Geometry: final body of the model. Coordinates: model frame, mm. Face numbers are marked on the shaded views. A direction names the side the tool comes from. Round coordinates to 2 decimals unless told otherwise and drop trailing zeros. Loops run counter-clockwise (first coordinate to the right, second up) from the corner with the lowest first, then second, coordinate; pieces in that order, holes last. Notation, with made-up numbers: (13, -20) - (62, -20) arc R20 cw to (62, 4) - close; hole circle Ø11 at (68.25, 36.5). An arc over 180 degrees is marked (long way). Answer as CSV lines item,"result".
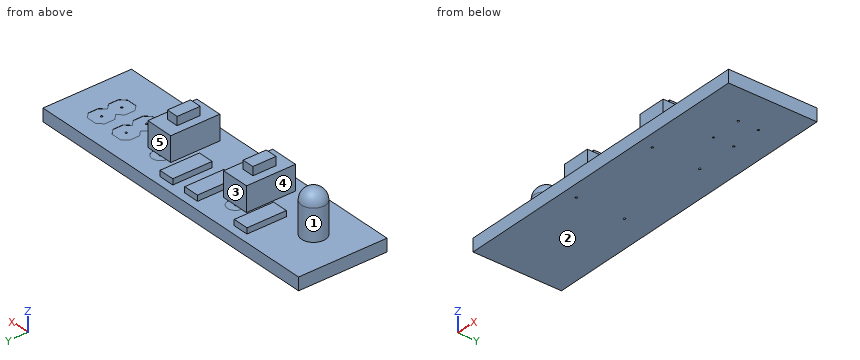
from build123d import *

# Parameters (mm, degrees)
SKETCH2_W           = 39.35
SKETCH2_H           = 11.1
BOSS_EXTRUDE1_DEPTH = 1.6
SKETCH3_W           = 1.966
SKETCH3_H           = 4.946
BOSS_EXTRUDE2_DEPTH = 0.72
SKETCH4_R           = 1.016
SKETCH4_R_2         = 0.13
CUT_EXTRUDE1_DEPTH  = 0.0254
SKETCH4_3_R         = 0.13
CUT_EXTRUDE2_DEPTH  = 41.916897487
CUT_EXTRUDE3_DEPTH  = 0.0254
SKETCH6_R           = 0.125
CUT_EXTRUDE4_DEPTH  = 41.915912127
SKETCH8_W           = 3.52
SKETCH8_H           = 6.16
BOSS_EXTRUDE3_DEPTH = 3.09
SKETCH9_W           = 1.5
SKETCH9_H           = 2.9
BOSS_EXTRUDE4_DEPTH = 1.07
LPATTERN1_COUNT     = 2
LPATTERN1_PITCH     = 11.668100108


with BuildPart() as part:
    # Sketch2 → Boss-Extrude1 (new body)
    with BuildSketch(Plane.XY):
        with Locations((19.675, 5.55)):
            Rectangle(SKETCH2_W, SKETCH2_H)
    extrude(amount=-BOSS_EXTRUDE1_DEPTH)

    # Sketch3 → Boss-Extrude2 (add)
    with BuildSketch(Plane.XY):
        with Locations((10.16, 7.62)):
            Rectangle(SKETCH3_W, SKETCH3_H)
        with Locations((17.78, 7.62)):
            Rectangle(SKETCH3_W, SKETCH3_H)
        with Locations((21.59, 7.62)):
            Rectangle(SKETCH3_W, SKETCH3_H)
    extrude(amount=BOSS_EXTRUDE2_DEPTH)

    # Sketch4 → Cut-Extrude1 (cut)
    # profile 1 of 8: a face of its own
    with BuildSketch(Plane.XY):
        with Locations((13.97, 1.5875)):
            Circle(SKETCH4_R)
        with Locations((13.97, 1.5875)):
            Circle(SKETCH4_R_2, mode=Mode.SUBTRACT)
    # profile 2 of 8: a face of its own
    with BuildSketch(Plane.XY):
        with Locations((13.97, 1.5875)):
            Circle(SKETCH4_R_2)
    # profile 3 of 8: a face of its own
    with BuildSketch(Plane.XY):
        with Locations((25.6381, 1.5875)):
            Circle(SKETCH4_R)
        with Locations((25.6381, 1.5875)):
            Circle(SKETCH4_R_2, mode=Mode.SUBTRACT)
    # profile 4 of 8: a face of its own
    with BuildSketch(Plane.XY):
        with Locations((25.6381, 1.5875)):
            Circle(SKETCH4_R_2)
    # profile 5 of 8: a face of its own
    with BuildSketch(Plane.XY):
        with Locations((25.5587, 7.62)):
            Circle(SKETCH4_R)
        with Locations((25.5587, 7.62)):
            Circle(SKETCH4_R_2, mode=Mode.SUBTRACT)
    # profile 6 of 8: a face of its own
    with BuildSketch(Plane.XY):
        with Locations((25.5587, 7.62)):
            Circle(SKETCH4_R_2)
    # profile 7 of 8: a face of its own
    with BuildSketch(Plane.XY):
        with Locations((13.97, 7.62)):
            Circle(SKETCH4_R)
        with Locations((13.97, 7.62)):
            Circle(SKETCH4_R_2, mode=Mode.SUBTRACT)
    # profile 8 of 8: a face of its own
    with BuildSketch(Plane.XY):
        with Locations((13.97, 7.62)):
            Circle(SKETCH4_R_2)
    extrude(amount=-CUT_EXTRUDE1_DEPTH, mode=Mode.SUBTRACT)

    # Sketch4_3 → Cut-Extrude2 (cut, through all)
    with BuildSketch(Plane.XY):
        with Locations((13.97, 1.5875)):
            Circle(SKETCH4_3_R)
        with Locations((25.6381, 1.5875)):
            Circle(SKETCH4_3_R)
        with Locations((25.5587, 7.62)):
            Circle(SKETCH4_3_R)
        with Locations((13.97, 7.62)):
            Circle(SKETCH4_3_R)
    extrude(amount=-CUT_EXTRUDE2_DEPTH, mode=Mode.SUBTRACT)

    # Sketch5 → Cut-Extrude3 (cut)
    with BuildSketch(Plane.XY):
        Polygon((29.5275, 6.985), (29.5275, 8.255), (30.1625, 8.89), (31.4325, 8.89), (32.0675, 8.255), (32.0675, 6.985), (31.4325, 6.35), (32.0675, 5.715), (32.0675, 4.445), (31.4325, 3.81), (30.1625, 3.81), (29.5275, 4.445), (29.5275, 5.715), (30.1625, 6.35), align=None)
        Polygon((33.3375, 4.445), (33.3375, 5.715), (33.9725, 6.35), (33.3375, 6.985), (33.3375, 8.255), (33.9725, 8.89), (35.2425, 8.89), (35.8775, 8.255), (35.8775, 6.985), (35.2425, 6.35), (35.8775, 5.715), (35.8775, 4.445), (35.2425, 3.81), (33.9725, 3.81), align=None)
    extrude(amount=-CUT_EXTRUDE3_DEPTH, mode=Mode.SUBTRACT)

    # Sketch6 → Cut-Extrude4 (cut, through all)
    with BuildSketch(Plane.XY.offset(-0.0254)):
        with Locations((30.7975, 7.62)):
            Circle(SKETCH6_R)
        with Locations(Location((30.7975, 5.08, 0), (0, 0, 180))):
            Circle(SKETCH6_R)
        with Locations((34.6075, 5.08)):
            Circle(SKETCH6_R)
        with Locations(Location((34.6075, 7.62, 0), (0, 0, 180))):
            Circle(SKETCH6_R)
    extrude(amount=-CUT_EXTRUDE4_DEPTH, mode=Mode.SUBTRACT)

    # Sketch8 → Boss-Extrude3 (add)
    with BuildSketch(Plane.XY):
        with Locations((13.97, 4.60375)):
            Rectangle(SKETCH8_W, SKETCH8_H)
    boss_extrude3 = extrude(amount=BOSS_EXTRUDE3_DEPTH)

    # Sketch9 → Boss-Extrude4 (add)
    with BuildSketch(Plane.XY.offset(3.09)):
        with Locations((13.97, 4.60375)):
            Rectangle(SKETCH9_W, SKETCH9_H)
    boss_extrude4 = extrude(amount=BOSS_EXTRUDE4_DEPTH)

    # LPattern1: Boss-Extrude3, Boss-Extrude4 ×2
    with Locations(*[(i * LPATTERN1_PITCH, 0, 0) for i in range(1, LPATTERN1_COUNT)]):
        add(boss_extrude3)
        add(boss_extrude4)

    # Sketch11 → Revolve18 (revolve)
    with BuildSketch(Plane.ZY.offset(-5.079644146), mode=Mode.PRIVATE) as revolve18_sk:
        with BuildLine():
            Line((0, 5.08), (0, 6.58))
            Line((0, 6.58), (3.95, 6.58))
            ThreePointArc((3.95, 6.58), (5.010660172, 6.140660172), (5.45, 5.08))
            Line((5.45, 5.08), (0, 5.08))
        make_face()
    revolve(revolve18_sk.sketch.rotate(Axis((5.079644146, 5.08, 0), (0, 0, 1)), 90), axis=Axis((5.079644146, 5.08, 0), (0, 0, 1)))


solid = part.part
(1) Pin query (flat end, axial travel): P1, Ø2, axis at x = 21.5, y = 6.5, coming from the +Z side; P2, Ø1.5, axis at y = 9.5, z = 2.5, coming from the -X side; P3, Ø0.9, axis at x = 26, z = 3.5, coming from the +Y side; P4, Ø0.9, axis at x = 25.5, z = 1, coming from the -Y side. Return the tip coordinate at first contact, or that it passes through.
Findings below:
P1,"z = 0.72"
P2,"through"
P3,"y = 7.68"
P4,"y = 1.52"
(2) Draft query along X for the marked faces 1 and 2. Return one class per face: pulls with the +X half, pulls with the -X half, needs draft (parallel to the pull), parting line crosses it, or undercut.
Findings below:
face 1,"undercut"
face 2,"needs draft"
(3) Section B-B (x = 23.5). Output: boundary loops of the cut face in (y, z), and give its area (3 significant figures).
Findings below:
outline,"(0, -1.6) - (11.1, -1.6) - (11.1, 0) - (0, 0) - close"
area,"17.8 mm2"
(4) Section A-A (z = 2.75). Output: boundary loops of the cut face in (x, y), and give its area (3 significant figures).
Findings below:
outline,"circle Ø3 at (5.08, 5.08); (12.21, 1.52) - (15.73, 1.52) - (15.73, 7.68) - (12.21, 7.68) - close; (23.88, 1.52) - (27.4, 1.52) - (27.4, 7.68) - (23.88, 7.68) - close"
area,"50.4 mm2"
(5) Material intervals for line 1 along X through (y, z) = (7.62, 0.05); line 2 along X through (y, z) = (9, 0.25); line 3 along X through (y, z) = (1.5, -0.25), sorted ascending.
Findings below:
line 1,"9.18 to 11.14, 12.21 to 15.73, 16.8 to 18.76, 20.61 to 22.57, 23.88 to 27.4"
line 2,"9.18 to 11.14, 16.8 to 18.76, 20.61 to 22.57"
line 3,"0 to 13.87, 14.07 to 25.54, 25.73 to 39.35"
(6) Access query for the marked faces 3, 4 and 5. Directions: +Z, -Z, +X, -X, +Y, -Y. A direction counts if a zero-diameter tool reaches every point of the face in a straight line with its end or side. Return the directions, or none.
Findings below:
face 3,"+Z, +Y"
face 4,"+Z, +Y, -Y"
face 5,"+Z, +X, +Y"
